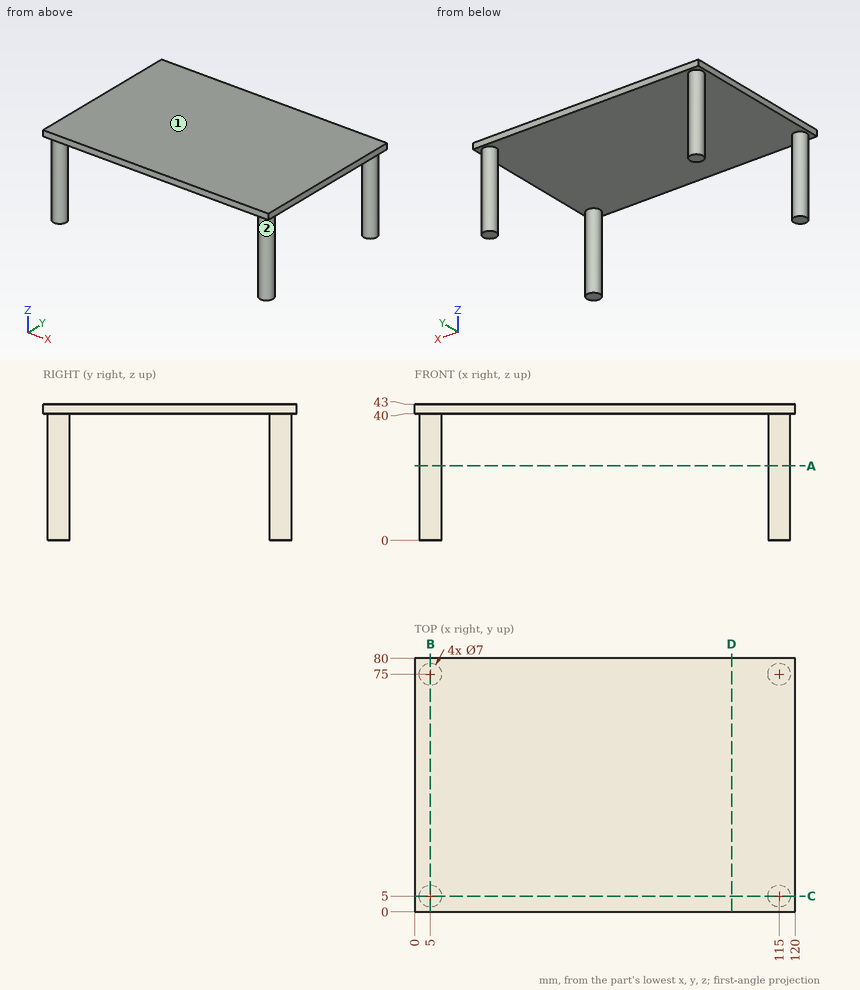
Geometry: see drawing. Coordinates: mm, zero at the bounding-box minimum. Coordinates: 2 decimals unless noted, no trailing zeros. Loops run counter-clockwise (first coordinate to the right, second up) from the corner with the lowest first, then second, coordinate; pieces in that order, holes last. Notation, with made-up numbers: M -12.75,-15.75 L 10.25,-15.75 A25 ccw 10.25,3.25 Z; hole C 21.5,8 d2. An arc over 180 degrees is marked long. Answer in a Markdown table with one row per item.
Q1. Ray query, probe 1 along Z at (x, y) = (95, 20.5); probe 2 along X at (y, z) = (6.5, 2.5); probe 3 along X at (y, z) = (73, 22). Return the intervals inside material, ascending. Write a range as from..to.
Answers below:
| item | result |
|---|---|
| probe 1 | z = 40..43 |
| probe 2 | x = 1.84..8.16, 111.84..118.16 |
| probe 3 | x = 2.13..7.87, 112.13..117.87 |
Q2. Draft query along X for the marked faces 1 and 2. Return one class per face: pulls with the +X half, pulls with the -X half, needs draft (parallel to the pull), parting line crosses it, or undercut.
Answers below:
| item | result |
|---|---|
| face 1 | needs draft |
| face 2 | undercut |
Q3. Section B-B on x = 5. Return the cut outline in (y, z).
Answers below:
| item | result |
|---|---|
| outline | M 0,40 L 1.5,40 L 1.5,0 L 8.5,0 L 8.5,40 L 71.5,40 L 71.5,0 L 78.5,0 L 78.5,40 L 80,40 L 80,43 L 0,43 Z |
Q4. Section A-A on z = 23.5. Return the cut outline in (x, y), plus the area to 3 significant figures.
Answers below:
| item | result |
|---|---|
| outline | C 5,5 d7; C 5,75 d7; C 115,5 d7; C 115,75 d7 |
| area | 154 mm^2 |
Q5. Section C-C on y = 5. Return the cut outline in (x, z).
Answers below:
| item | result |
|---|---|
| outline | M 0,40 L 1.5,40 L 1.5,0 L 8.5,0 L 8.5,40 L 111.5,40 L 111.5,0 L 118.5,0 L 118.5,40 L 120,40 L 120,43 L 0,43 Z |
Q6. Section D-D on x = 100. Return the cut outline in (y, z).
Answers below:
| item | result |
|---|---|
| outline | M 0,40 L 80,40 L 80,43 L 0,43 Z |
Q7. First-contact query: pin 1 (24 mm diameter, centred on x = 43, y = 54, fed in from -Z). Flat tip, straight axial feed; report the tip coordinate or a pass-through.
Answers below:
| item | result |
|---|---|
| pin 1 | stops at z = 40 |
